from build123d import *

# Parameters (mm, degrees)
SKETCH1_R           = 6.5
BOSS_EXTRUDE1_DEPTH = 3
SKETCH2_W           = 30
SKETCH2_H           = 2.5
BOSS_EXTRUDE2_DEPTH = 8.5
FILLET1_R           = 1
SKETCH3_R           = 1.5
CUT_EXTRUDE1_DEPTH  = 8.5


with BuildPart() as part:
    # Sketch1 → Boss-Extrude1 (new body)
    with BuildSketch(Plane(origin=(0, 0, 0), x_dir=(1, 0, 0), z_dir=(0, 1, 0))):
        with BuildLine():
            Line((-15, 0), (15, 0))
            Line((15, 0), (15, -2.5))
            Line((15, -2.5), (10.523048028, -17.203975688))
            ThreePointArc((10.523048028, -17.203975688), (0, -25), (-10.523048028, -17.203975688))
            Line((-10.523048028, -17.203975688), (-15, -2.5))
            Line((-15, -2.5), (-15, 0))
        make_face()
        with Locations(Location((0, -14, 0), (0, 0, 270))):
            Circle(SKETCH1_R, mode=Mode.SUBTRACT)
    extrude(amount=-BOSS_EXTRUDE1_DEPTH)

    # Sketch2 → Boss-Extrude2 (add)
    with BuildSketch(Plane(origin=(0, 0, 0), x_dir=(1, 0, 0), z_dir=(0, 1, 0))):
        with Locations((0, -1.25)):
            Rectangle(SKETCH2_W, SKETCH2_H)
    extrude(amount=BOSS_EXTRUDE2_DEPTH)

    # Fillet1
    fillet1_edges = [part.edges().sort_by_distance(p)[0] for p in [
        (-15, 8.5, 1.25),
        (15, 8.5, 1.25),
    ]]
    fillet(fillet1_edges, radius=FILLET1_R)

    # Sketch3 → Cut-Extrude1 (cut)
    with BuildSketch(Plane.XY.offset(2.5)):
        with Locations((11.5, 5.874642398)):
            Circle(SKETCH3_R)
    cut_extrude1 = extrude(amount=-CUT_EXTRUDE1_DEPTH, mode=Mode.SUBTRACT)

    # Mirror1: Cut-Extrude1 across plane
    add(cut_extrude1.mirror(Plane(origin=(0, 0, 0), x_dir=(0, 0, 1), z_dir=(1, 0, 0))), mode=Mode.SUBTRACT)


solid = part.part
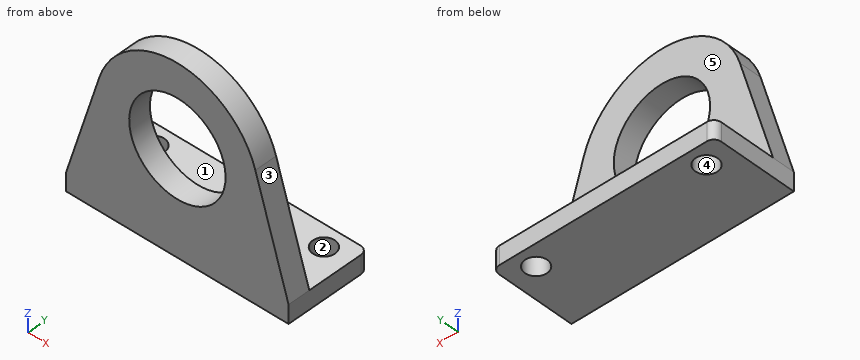
Geometry: final body of the model. Coordinates: model frame, mm. Face numbers are marked on the shaded views. A direction names the side the tool comes from. Round coordinates to 2 decimals unless told otherwise and drop trailing zeros. Loops run counter-clockwise (first coordinate to the right, second up) from the corner with the lowest first, then second, coordinate; pieces in that order, holes last. Notation, with made-up numbers: (-10, 18) -> (13, 18) arc R16 cw to (13, 48) -> close; hole circle Ø11 at (-15.5, 57). An arc over 180 degrees is marked (long way). One line per question, with ' | ' between items. Start each with the question number.
1. Section B-B on x = 0. Output: boundary loops of the cut face in (y, z).
2. Contact query for flat-ended pins moving along their axis: pin 1 (12 mm diameter, centred on x = -11.5, z = 12.5, fed in from +Y); pin 2 (4 mm diameter, centred on x = 11.5, y = 5.87, fed in from +Z). Output: stop coordinate, or through.
3. Section D-D on y = 6.25. Output: boundary loops of the cut face in (x, z).
4. Line query: line 1 along Y through (x, z) = (11.5, 0.95); line 2 along Y through (x, z) = (10.5, 11.75); line 3 along Z through (x, y) = (4.75, 6). Output: solid intervals per line, ascending. Write a range as [from, to].
5. Section A-A on y = -1. Output: boundary loops of the cut face in (x, z), and give its area (3 significant figures).
6. Set-up query: the marked faces 4 and 5. Return all of +Z, -Z, +X, -X, +Y, -Y with unobstructed straight access to the full face (end or side cutting, diameter ignored); none if empty.
7. Section C-C on z = 11.25. Output: boundary loops of the cut face in (x, y), and give its area (3 significant figures).
8. Mould query, pull axis X, two halves, no side actions, for the marked faces 1, 2 and 3. Classes: pulls with the +X half, pulls with the -X half, needs draft (parallel to the pull), parting line crosses it, or undercut.
Returned:
1) outline: (-3, 0) -> (8.5, 0) -> (8.5, 2.5) -> (0, 2.5) -> (0, 7.5) -> (-3, 7.5) -> close; (-3, 20.5) -> (0, 20.5) -> (0, 25) -> (-3, 25) -> close
2) pin 1: stops at y = 0 | pin 2: stops at z = 2.5
3) outline: (-15, 0) -> (-12.95, 0) -> (-12.95, 2.5) -> (-15, 2.5) -> close; (-10.05, 0) -> (10.05, 0) -> (10.05, 2.5) -> (-10.05, 2.5) -> close; (12.95, 0) -> (15, 0) -> (15, 2.5) -> (12.95, 2.5) -> close
4) line 1: y = [-3, 4.37], [7.37, 8.5] | line 2: y = [-3, 0] | line 3: z = [0, 2.5]
5) outline: (-15, 0) -> (15, 0) -> (15, 2.5) -> (10.52, 17.2) arc R11 ccw to (-10.52, 17.2) -> (-15, 2.5) -> close; hole circle Ø13 at (0, 14) | area: 438 mm2
6) face 4: +Z, -Z | face 5: +Z, +X, -X, +Y
7) outline: (-12.34, -3) -> (-5.89, -3) -> (-5.89, 0) -> (-12.34, 0) -> close; (5.89, -3) -> (12.34, -3) -> (12.34, 0) -> (5.89, 0) -> close | area: 38.7 mm2
8) face 1: needs draft | face 2: undercut | face 3: pulls with the +X half
